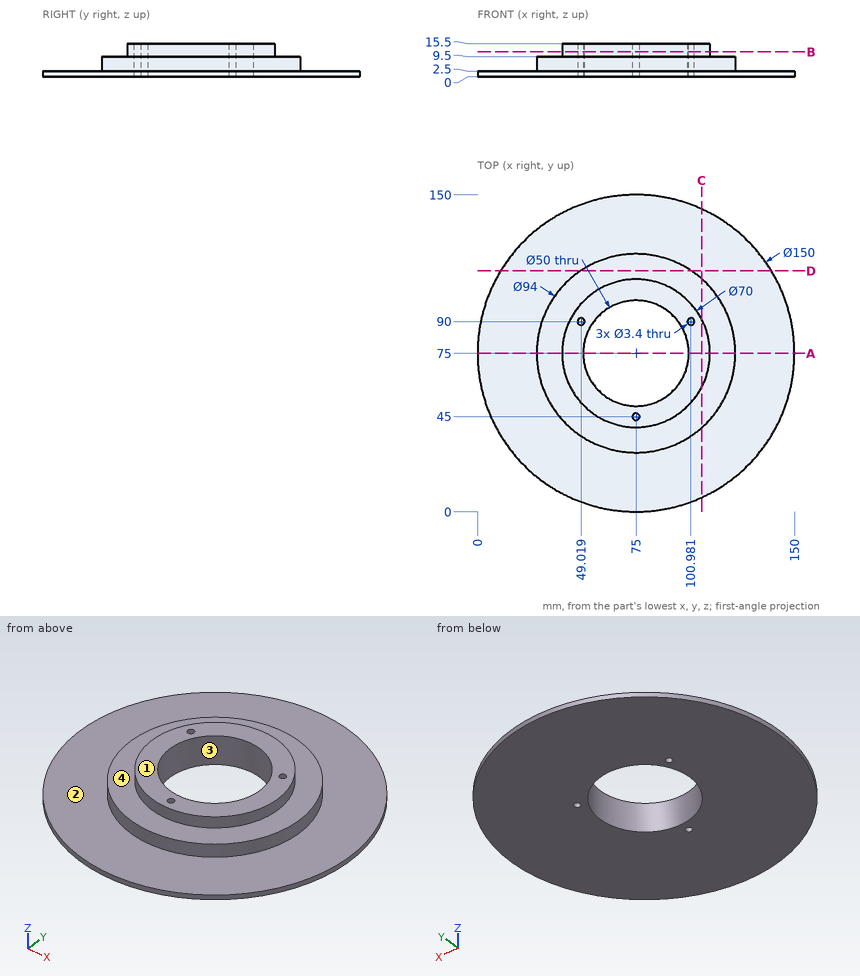
Study the drawing (mm; zero at the part's minimum x, y, z) and answer. A direction names the side the tool comes from. Coordinates: 2 decimals unless noted, no trailing zeros. Order: outer loops, then holes, each group sorted by start corner. A loop starts at its lowest first (then second) coordinate and runs counter-clockwise, first axis right, second up. Notation, with made-up numbers: (-35.5, 19) -> (12.5, 19) arc R27 ccw to (12.5, 49) -> close; hole circle Ø4 at (-39.75, -22.75). An arc over 180 degrees is marked (long way). Answer in a Markdown table with one row per item. Add a question column.
Item 1: Find section B-B (z = 11.75). Write down the section's boundary in (x, y), then the cut area to 3 significant figures.
Item 2: Find section D-D (y = 114). Write down the section's boundary in (x, z).
Item 3: Find section C-C (x = 106). Write down the section's boundary in (y, z).
Item 4: Which of the six approach directions +Z, -Z, +X, -X, +Y, -Y give full straight-line access (tool end or side, diameter ignored) to the marked faces 1 and 2?
Item 5: Each of these flat-tipped pins is pushed along its axis until it touches: P1, Ø6, axis at y = 83.5, z = 9.5, coming from the +X side; P2, Ø1.5, axis at y = 33, z = 4.5, coming from the +X side (1 decimal); P3, Ø1, axis at y = 120, z = 11.5, coming from the -X side. Where does it stop, or does it pass through?
Item 6: Find section A-A (y = 75). Write down the section's boundary in (x, z).
Item 7: Find the intervals of material crossed by L1, parallel to Y at x = 73.5, z = 14 (1 decimal); L2, parallel to X at y = 90, z = 3.75; L3, parallel to Y at x = 75, z = 7.25, in increasing order. Write a range as from..to.
Item 8: Determine the mould class of the marked faces 3 and 4 for opening direction Y: +Y half, -Y half, draft (parallel to the pull), parting line (faces both ways), or undercut.
Result set:
| question | item | result |
|---|---|---|
| 1 | outline | circle Ø70 at (75, 75); hole circle Ø3.4 at (49.02, 90); hole circle Ø50 at (75, 75); hole circle Ø3.4 at (75, 45); hole circle Ø3.4 at (100.98, 90) |
| 1 | area | 1,860 mm² |
| 2 | outline | (10.94, 0) -> (139.06, 0) -> (139.06, 2.5) -> (101.23, 2.5) -> (101.23, 9.5) -> (48.77, 9.5) -> (48.77, 2.5) -> (10.94, 2.5) -> close |
| 3 | outline | (6.71, 0) -> (143.29, 0) -> (143.29, 2.5) -> (110.33, 2.5) -> (110.33, 9.5) -> (91.25, 9.5) -> (91.25, 15.5) -> (58.75, 15.5) -> (58.75, 9.5) -> (39.67, 9.5) -> (39.67, 2.5) -> (6.71, 2.5) -> close |
| 4 | face 1 | +Z, +X, -X, +Y, -Y |
| 4 | face 2 | +Z |
| 5 | P1 | stops at x = 121.68 |
| 5 | P2 | stops at x = 97.5 |
| 5 | P3 | passes through |
| 6 | outline | (0, 0) -> (50, 0) -> (50, 15.5) -> (40, 15.5) -> (40, 9.5) -> (28, 9.5) -> (28, 2.5) -> (0, 2.5) -> close; (100, 0) -> (150, 0) -> (150, 2.5) -> (122, 2.5) -> (122, 9.5) -> (110, 9.5) -> (110, 15.5) -> (100, 15.5) -> close |
| 7 | L1 | y = 40..44.2, 45.8..50, 100..110 |
| 7 | L2 | x = 30.46..47.32, 50.72..55, 95..99.28, 102.68..119.54 |
| 7 | L3 | y = 28..43.3, 46.7..50, 100..122 |
| 8 | face 3 | undercut |
| 8 | face 4 | draft |
